```python
from build123d import *

# Parameters (mm, degrees)
SKETCH1_W           = 46
SKETCH1_H           = 36
SKETCH1_W_2         = 42
SKETCH1_H_2         = 32
BOSS_EXTRUDE1_DEPTH = 55
SKETCH2_W           = 42
SKETCH2_H           = 32
BOSS_EXTRUDE2_DEPTH = 5
FILLET1_R           = 2.5
BOSS_EXTRUDE3_DEPTH = 10
SKETCH3_W           = 25
SKETCH3_H           = 15
CUT_EXTRUDE1_DEPTH  = 47
SKETCH5_W           = 35
SKETCH5_H           = 15
CUT_EXTRUDE2_DEPTH  = 37
CUT_EXTRUDE3_REACH  = 7
SKETCH7_R           = 3.25


with BuildPart() as part:
    # Sketch1 → Boss-Extrude1 (new body)
    with BuildSketch(Plane(origin=(0, 0, 0), x_dir=(1, 0, 0), z_dir=(0, 1, 0))):
        Rectangle(SKETCH1_W, SKETCH1_H)
        Rectangle(SKETCH1_W_2, SKETCH1_H_2, mode=Mode.SUBTRACT)
    extrude(amount=BOSS_EXTRUDE1_DEPTH)

    # Sketch2 → Boss-Extrude2 (add)
    with BuildSketch(Plane.XZ):
        Rectangle(SKETCH2_W, SKETCH2_H)
    extrude(amount=-BOSS_EXTRUDE2_DEPTH)

    # Fillet1
    fillet1_edges = [part.edges().sort_by_distance(p)[0] for p in [
        (-23, 27.5, -18),
        (23, 27.5, -18),
        (23, 27.5, 18),
        (-23, 27.5, 18),
    ]]
    fillet(fillet1_edges, radius=FILLET1_R)

    # Sketch4 → Boss-Extrude3 (add)
    with BuildSketch(Plane(origin=(0, 5, 0), x_dir=(1, 0, 0), z_dir=(0, 1, 0))):
        with BuildLine():
            Line((-21, -16), (-13.5, -16))
            ThreePointArc((-13.5, -16), (-15.696699141, -10.696699141), (-21, -8.5))
            Line((-21, -8.5), (-21, -16))
        make_face()
        with BuildLine():
            Line((21, 16), (13.5, 16))
            ThreePointArc((13.5, 16), (15.696699141, 10.696699141), (21, 8.5))
            Line((21, 8.5), (21, 16))
        make_face()
    extrude(amount=BOSS_EXTRUDE3_DEPTH)

    # Sketch3 → Cut-Extrude1 (cut, through all)
    with BuildSketch(Plane(origin=(23, 0, -5), x_dir=(0, 0, 1), z_dir=(-1, 0, 0))):
        with Locations((5, 22.5)):
            Rectangle(SKETCH3_W, SKETCH3_H)
    extrude(amount=CUT_EXTRUDE1_DEPTH, mode=Mode.SUBTRACT)

    # Sketch5 → Cut-Extrude2 (cut, through all)
    with BuildSketch(Plane.XY.offset(18)):
        with Locations((0, 22.5)):
            Rectangle(SKETCH5_W, SKETCH5_H)
    extrude(amount=-CUT_EXTRUDE2_DEPTH, mode=Mode.SUBTRACT)

    # Sketch7 → Cut-Extrude3 (cut, up to next)
    with BuildSketch(Plane(origin=(0, 5, 0), x_dir=(1, 0, 0), z_dir=(0, 1, 0)), mode=Mode.PRIVATE) as cut_extrude3_sk1:
        Circle(SKETCH7_R)
    cut_extrude3_tool1 = extrude(cut_extrude3_sk1.sketch, amount=-CUT_EXTRUDE3_REACH, mode=Mode.PRIVATE) & part.part
    add(cut_extrude3_tool1.solids().sort_by_distance((0, 5, 0))[0], mode=Mode.SUBTRACT)


solid = part.part
```
Model file for the job. Use its own axes, mm. A direction names the side the tool comes from. Coordinates: 2 decimals unless noted, no trailing zeros. Order: outer loops, then holes, each group sorted by start corner. A loop starts at its lowest first (then second) coordinate and runs counter-clockwise, first axis right, second up. Notation, with made-up numbers: (-18, -12.5) -> (20, -12.5) arc R20 ccw to (20, 14.5) -> close; hole circle Ø6 at (89.5, -3.5). An arc over 180 degrees is marked (long way). Answer as a JSON object with one key per item and string values. Group by question number.
1) Cut at C-C, the plane y = 25. Write the cut outline in (x, z).
2) Cut at D-D, the plane z = 0. Write the cut outline in (x, y).
3) Pull direction Z, two halves, no side cores. Call faces 6 (the face through (-22, 22, -12.5)), 7 (the face through (-22.287, 27.885, -17.248)), 8 (the face through (17.5, 22, -17)), 9 (the face through (22, 30, 0)): +Z half, -Z half, draft (parallel to the pull), parting line (faces both ways), or undercut.
4) Flat gauge pins, fed straight in: pin 1 (3 mm diameter, centred on x = -9, z = -6.5, fed in from +Y); pin 2 (1.6 mm diameter, centred on y = 25, z = 17.5, fed in from -X); pin 3 (0.6 mm diameter, centred on y = 22, z = 16.5, fed in from +X). Where does each tip first touch, or does it go through?
5) Cut at B-B, the plane x = -9. Write the cut outline in (y, z), then the cut area to 3 significant figures.
6) Cut at A-A, the plane z = 6. Write the cut outline in (x, y).
7) Which spindle directions (+Z, -Z, +X, -X, +Y, -Y) get a long thin tool onto all of the face, cutting with end or side? Do faces 1 (the face through (10.3, 15, -16.4)), 2 (the face through (22, 22, 12.5)), 3 (the face through (0, 35, 16)), 4 (the face through (0, 30, 17)), 5 (the face through (22.248, 27.885, 17.287)). Say none if no direction does.
8) Drill centre lines: L1, parallel to X at y = 3.4, z = 0; L2, parallel to X at y = 49, z = -10; L3, parallel to Z at x = 9.5, y = 33.5. Where is each one in solid material? Low to high.
Check values:
{
 "1": {"outline": "(-23, -15.5) arc R2.5 ccw to (-20.5, -18) -> (-17.5, -18) -> (-17.5, -16) -> (-21, -16) -> (-21, -12.5) -> (-23, -12.5) -> close; (-23, 12.5) -> (-21, 12.5) -> (-21, 16) -> (-17.5, 16) -> (-17.5, 18) -> (-20.5, 18) arc R2.5 ccw to (-23, 15.5) -> close; (17.5, -18) -> (20.5, -18) arc R2.5 ccw to (23, -15.5) -> (23, -12.5) -> (21, -12.5) -> (21, -16) -> (17.5, -16) -> close; (17.5, 16) -> (21, 16) -> (21, 12.5) -> (23, 12.5) -> (23, 15.5) arc R2.5 ccw to (20.5, 18) -> (17.5, 18) -> close"},
 "2": {"outline": "(-23, 0) -> (-3.25, 0) -> (-3.25, 5) -> (-21, 5) -> (-21, 15) -> (-23, 15) -> close; (-23, 30) -> (-21, 30) -> (-21, 55) -> (-23, 55) -> close; (3.25, 0) -> (23, 0) -> (23, 15) -> (21, 15) -> (21, 5) -> (3.25, 5) -> close; (21, 30) -> (23, 30) -> (23, 55) -> (21, 55) -> close"},
 "3": {"face 6": "undercut", "face 7": "-Z half", "face 8": "draft", "face 9": "undercut"},
 "4": {"pin 1": "stops at y = 5", "pin 2": "stops at x = -22.69", "pin 3": "stops at x = 22.9"},
 "5": {"outline": "(0, -18) -> (15, -18) -> (15, -16) -> (5, -16) -> (5, 16) -> (15, 16) -> (15, 18) -> (0, 18) -> close; (30, -18) -> (55, -18) -> (55, -16) -> (30, -16) -> close; (30, 16) -> (55, 16) -> (55, 18) -> (30, 18) -> close", "area": "320 mm²"},
 "6": {"outline": "(-23, 0) -> (23, 0) -> (23, 15) -> (21, 15) -> (21, 5) -> (-21, 5) -> (-21, 15) -> (-23, 15) -> close; (-23, 30) -> (-21, 30) -> (-21, 55) -> (-23, 55) -> close; (21, 30) -> (23, 30) -> (23, 55) -> (21, 55) -> close"},
 "7": {"face 1": "none", "face 2": "+X, -X", "face 3": "+Y", "face 4": "+Z, -Z", "face 5": "+Z, +X, +Y, -Y"},
 "8": {"L1": "x = -23 to -3.25, 3.25 to 23", "L2": "x = -23 to -21, 21 to 23", "L3": "z = -18 to -16, 16 to 18"}
}
